from build123d import *

# Parameters (mm, degrees)
SKETCH1_R           = 9.5
BOSS_EXTRUDE1_DEPTH = 25
SKETCH2_R           = 2
CUT_EXTRUDE1_DEPTH  = 26
SKETCH3_R           = 5
CUT_EXTRUDE2_DEPTH  = 12.5


with BuildPart() as part:
    # Sketch1 → Boss-Extrude1 (new body)
    with BuildSketch(Plane.XY):
        Circle(SKETCH1_R)
    extrude(amount=BOSS_EXTRUDE1_DEPTH)

    # Sketch2 → Cut-Extrude1 (cut, through all)
    with BuildSketch(Plane.XY.offset(25)):
        Circle(SKETCH2_R)
    extrude(amount=-CUT_EXTRUDE1_DEPTH, mode=Mode.SUBTRACT)

    # Sketch3 → Cut-Extrude2 (cut)
    with BuildSketch(Plane(origin=(0, 0, 0), x_dir=(-1, 0, 0), z_dir=(0, 0, -1))):
        Circle(SKETCH3_R)
    extrude(amount=-CUT_EXTRUDE2_DEPTH, mode=Mode.SUBTRACT)


solid = part.part
Work out the finished part from the listing and answer in its coordinate system (mm). A direction names the side the tool comes from. Round coordinates to 2 decimals unless told otherwise and drop trailing zeros. Order: outer loops, then holes, each group sorted by start corner. A loop starts at its lowest first (then second) coordinate and runs counter-clockwise, first axis right, second up. Notation, with made-up numbers: M 66.5,22.5 L 88.5,22.5 A18 ccw 88.5,36.5 Z; hole C -16,25.5 d7. An arc over 180 degrees is marked long. Put each result on its own line as item: value. Start each with the question number.
Q1. Flat-ended cylindrical pins translate along their axes: pin 1 (3 mm diameter, centred on x = 0, y = 0, fed in from +Z); pin 2 (3 mm diameter, centred on y = -4, z = 5, fed in from +X); pin 3 (1 mm diameter, centred on y = -4, z = 5, fed in from -X); pin 4 (3 mm diameter, centred on x = -1, y = 1, fed in from -Z). Find the tip coordinate at first contact, or state that the pin passes through.
Q2. A tool of negligible diameter and unlimited length cuts with its end or side. For faces 1 (the flat face through (-0.1, 2.2, 25)), 2 (the flat face through (0.1, -2.2, 12.5)), from which of +Z, -Z, +X, -X, +Y, -Y can it reach the whole face along a straight path? Write none if from no direction.
Q3. For a pull along Y with two mould halves and no side action, classify faces 3 (the cylindrical face through (4.38, -8.43, 12.32)), 4 (the cylindrical face through (1.08, -4.88, 6.16)), 5 (the flat face through (4, -4, 0)) as pulls with the +Y half, pulls with the -Y half, needs draft (parallel to the pull), parting line crosses it, or undercut.
Q4. Straight lines are drawn through the part: L1, parallel to Y at x = 0, z = 2.5; L2, parallel to Y at x = 0, z = 16; L3, parallel to Z at x = 3, y = 0. For each, find the intervals that lie inside material, in ascending order. Write a range as [from, to].
Q5. Section A-A, the plane y = 0 is taken. Write down the section's boundary in (x, z), and give its area (3 significant figures).
Q6. Section D-D, the plane z = 9.25 is taken. Write down the section's boundary in (x, y).
Q7. Section C-C, the plane z = 15.5 is taken. Write down the section's boundary in (x, y), and give its area (3 significant figures).
Findings below:
1. pin 1: passes through
1. pin 2: stops at x = 9.17
1. pin 3: stops at x = -8.83
1. pin 4: stops at z = 12.5
2. face 1: +Z, +X, -X, +Y, -Y
2. face 2: -Z
3. face 3: parting line crosses it
3. face 4: undercut
3. face 5: needs draft
4. L1: y = [-9.5, -5], [5, 9.5]
4. L2: y = [-9.5, -2], [2, 9.5]
4. L3: z = [12.5, 25]
5. outline: M -9.5,0 L -5,0 L -5,12.5 L -2,12.5 L -2,25 L -9.5,25 Z; M 2,12.5 L 5,12.5 L 5,0 L 9.5,0 L 9.5,25 L 2,25 Z
5. area: 300 mm^2
6. outline: C 0,0 d19; hole C 0,0 d10
7. outline: C 0,0 d19; hole C 0,0 d4
7. area: 271 mm^2
